Can you work these out from the model? Positions are in its coordinate system, mm. A direction names the side the tool comes from. Coordinates: 2 decimals unless noted, no trailing zeros. Order: outer loops, then holes, each group sorted by start corner. A loop starts at its lowest first (then second) coordinate and runs counter-clockwise, first axis right, second up. Notation, with made-up numbers: (-29, 33) -> (-7, 33) arc R16 ccw to (-7, 39) -> close; hole circle Ø8 at (-35, 42). An arc over 180 degrees is marked (long way). Answer as CSV lines item,"result".
from build123d import *

# Parameters (mm, degrees)
ESQUISSE1_R                                 = 30
BOSS_EXTRU_1_DEPTH                          = 10
CHANFREIN1_SIZE                             = 10
CHANFREIN1_SIZE_2                           = 7.002075382
COQUE2_T                                    = -1.5
ESQUISSE2_R                                 = 4.000000000000001
BOSS_EXTRU_2_DEPTH                          = 8.5
CHANFREIN2_SIZE                             = 8.5
CHANFREIN2_SIZE_2                           = 0.445466124
ESQUISSE5_R                                 = 2.5545338760941463
ENL_V_MAT_EXTRU_1_DEPTH                     = 10
R_P_TITION_CIRCULAIRE1_COUNT                = 3
CHANFREIN2_OF_R_P_TITION_CIRCULAIRE1_SIZE   = 0.445466124
CHANFREIN2_OF_R_P_TITION_CIRCULAIRE1_SIZE_2 = 8.5
ESQUISSE6_R                                 = 8.5
ENL_V_MAT_EXTRU_2_DEPTH                     = 8.5


with BuildPart() as part:
    # Esquisse1 → Boss.-Extru.1 (new body)
    with BuildSketch(Plane(origin=(0, 0, 0), x_dir=(1, 0, 0), z_dir=(0, 1, 0))):
        with Locations(Location((0, 0, 0), (0, 0, 270))):
            Circle(ESQUISSE1_R)
    extrude(amount=BOSS_EXTRU_1_DEPTH)

    # Chanfrein1
    # the kernel refuses this chamfer: 10, 7.002075382 mm, written as the material it takes off along each edge
    with BuildSketch(Plane(origin=(0, 10, 0), x_dir=(-1.8e-16, 0, 1), z_dir=(-1, 0, -1.8e-16))) as chanfrein1_piece_1:
        Polygon((30, -CHANFREIN1_SIZE), (30 - CHANFREIN1_SIZE_2, 0), (30, 0), align=None)
    revolve(axis=Axis((0, 10, 0), (0, 1, 0)), mode=Mode.SUBTRACT)

    # Coque2
    coque2_openings = [part.faces().sort_by_distance(p)[0] for p in [
        (0, 0, 0),
    ]]
    offset(amount=COQUE2_T, openings=coque2_openings, kind=Kind.INTERSECTION)

    # Esquisse2 → Boss.-Extru.2 (add)
    with BuildSketch(Plane.XZ.offset(-8.5)):
        with Locations(Location((-16, 0, 0), (0, 0, 90))):
            Circle(ESQUISSE2_R)
    boss_extru_2 = extrude(amount=BOSS_EXTRU_2_DEPTH)

    # Chanfrein2
    # the kernel refuses this chamfer: 8.5, 0.445466124 mm, written as the material it takes off along each edge
    with BuildSketch(Plane(origin=(-16, 0, 0), x_dir=(0, 0, 1), z_dir=(1, 0, 0))) as chanfrein2_piece_1_section:
        Polygon((4.000000000000001, -CHANFREIN2_SIZE), (4.000000000000001 - CHANFREIN2_SIZE_2, 0), (4.000000000000001, 0), align=None)
    chanfrein2_piece_1 = revolve(axis=Axis((-16, 0, 0), (0, -1, 0)), mode=Mode.PRIVATE)
    chanfrein2_piece_1 = split(chanfrein2_piece_1, bisect_by=Plane(origin=(-16, 8.5, -3.8124488578332274), z_dir=(0, -1, 0)), keep=Keep.TOP, mode=Mode.PRIVATE)
    add(chanfrein2_piece_1, mode=Mode.SUBTRACT)

    # Esquisse5 → Enlèv. mat.-Extru.1 (cut)
    with BuildSketch(Plane.XZ):
        with Locations(Location((-16, 0, 0), (0, 0, 270))):
            Circle(ESQUISSE5_R)
    enl_v_mat_extru_1 = extrude(amount=-ENL_V_MAT_EXTRU_1_DEPTH, mode=Mode.SUBTRACT)

    # Répétition circulaire1: Boss.-Extru.2, Enlèv. mat.-Extru.1 ×3 about axis
    r_p_tition_circulaire1_axis = Axis((9.3e-16, 0, 6.2e-16), (0, 1, 0))
    add([boss_extru_2.rotate(r_p_tition_circulaire1_axis, i * 360 / R_P_TITION_CIRCULAIRE1_COUNT) for i in range(1, R_P_TITION_CIRCULAIRE1_COUNT)])
    add([enl_v_mat_extru_1.rotate(r_p_tition_circulaire1_axis, i * 360 / R_P_TITION_CIRCULAIRE1_COUNT) for i in range(1, R_P_TITION_CIRCULAIRE1_COUNT)], mode=Mode.SUBTRACT)

    # Chanfrein2 of Répétition circulaire1
    # the kernel refuses this chamfer: 8.5, 0.445466124 mm, written as the material it takes off along each edge
    with BuildSketch(Plane(origin=(7.999999999999997, 0, 13.856406460551021), x_dir=(0.8660254037844387, 0, -0.5000000000000001), z_dir=(-0.5000000000000001, 0, -0.8660254037844387))) as chanfrein2_of_r_p_tition_circulaire1_piece_1_section:
        Polygon((4 - CHANFREIN2_OF_R_P_TITION_CIRCULAIRE1_SIZE, 0), (4.000000000000002, -CHANFREIN2_OF_R_P_TITION_CIRCULAIRE1_SIZE_2), (4, 0), align=None)
    chanfrein2_of_r_p_tition_circulaire1_piece_1 = revolve(axis=Axis((7.999999999999997, 0, 13.856406460551021), (0, -1, 0)), mode=Mode.PRIVATE)
    chanfrein2_of_r_p_tition_circulaire1_piece_1 = split(chanfrein2_of_r_p_tition_circulaire1_piece_1, bisect_by=Plane(origin=(4.6983224384874545, 8.5, 15.762630889467637), z_dir=(0, -1, 0)), keep=Keep.TOP, mode=Mode.PRIVATE)
    add(chanfrein2_of_r_p_tition_circulaire1_piece_1, mode=Mode.SUBTRACT)
    with BuildSketch(Plane(origin=(8.000000000000009, 0, -13.856406460551014), x_dir=(-0.8660254037844384, 0, -0.5000000000000003), z_dir=(-0.5000000000000003, 0, 0.8660254037844384))) as chanfrein2_of_r_p_tition_circulaire1_piece_2_section:
        Polygon((4 - CHANFREIN2_OF_R_P_TITION_CIRCULAIRE1_SIZE, 0), (4, -CHANFREIN2_OF_R_P_TITION_CIRCULAIRE1_SIZE_2), (4, 0), align=None)
    chanfrein2_of_r_p_tition_circulaire1_piece_2 = revolve(axis=Axis((8.000000000000009, 0, -13.856406460551014), (0, -1, 0)), mode=Mode.PRIVATE)
    chanfrein2_of_r_p_tition_circulaire1_piece_2 = split(chanfrein2_of_r_p_tition_circulaire1_piece_2, bisect_by=Plane(origin=(11.301677561512552, 8.5, -11.950182031634398), z_dir=(0, -1, 0)), keep=Keep.TOP, mode=Mode.PRIVATE)
    add(chanfrein2_of_r_p_tition_circulaire1_piece_2, mode=Mode.SUBTRACT)

    # Esquisse6 → Enlèv. mat.-Extru.2 (cut)
    with BuildSketch(Plane.XZ.offset(-8.5)):
        with Locations(Location((0, 0, 0), (0, 0, 270))):
            Circle(ESQUISSE6_R)
    extrude(amount=-ENL_V_MAT_EXTRU_2_DEPTH, mode=Mode.SUBTRACT)


solid = part.part
Q1. We'd pull the mould along Z, two halves only. Please class faces 1 (the conical face through (-12.65, 4.19, 1.74)), 2 (the flat face through (0, 10, 10)), 3 (the conical face through (7.01, 9.514, 22.26)): pulls with the +Z half, pulls with the -Z half, needs draft (parallel to the pull), parting line crosses it, or undercut.
Solution:
face 1,"undercut"
face 2,"needs draft"
face 3,"parting line crosses it"
Q2. Imagine slicing it at A-A (x = 0). List the corners of the cut face in (y, z) for me, and give its area (3 significant figures).
Solution:
outline,"(0, -30) -> (10, -23) -> (10, -8.5) -> (8.5, -8.5) -> (8.5, -22.22) -> (0, -28.17) -> close; (0, 28.17) -> (8.5, 22.22) -> (8.5, 8.5) -> (10, 8.5) -> (10, 23) -> (0, 30) -> close"
area,"76.2 mm2"
Q3. Imagine slicing it at C-C (y = 4.25). List the corners of the cut face in (x, z) for me, and give its area (3 significant figures).
Solution:
outline,"circle Ø54.05 at (0, 0); circle Ø7.55 at (-16, 0); circle Ø7.55 at (8, -13.86); circle Ø7.55 at (8, 13.86); hole circle Ø50.39 at (0, 0); hole circle Ø5.11 at (-16, 0); hole circle Ø5.11 at (8, -13.86); hole circle Ø5.11 at (8, 13.86)"
area,"373 mm2"
Q4. Imagine slicing it at D-D (y = 0.75). List the corners of the cut face in (x, z) for me, and give its area (3 significant figures).
Solution:
outline,"circle Ø58.95 at (0, 0); circle Ø7.19 at (-16, 0); circle Ø7.19 at (8, -13.86); circle Ø7.19 at (8, 13.86); hole circle Ø55.29 at (0, 0); hole circle Ø5.11 at (-16, 0); hole circle Ø5.11 at (8, -13.86); hole circle Ø5.11 at (8, 13.86)"
area,"389 mm2"
Q5. Imagine slicing it at B-B (z = 0). List the corners of the cut face in (x, y) for me, and give its area (3 significant figures).
Solution:
outline,"(-30, 0) -> (-28.17, 0) -> (-22.22, 8.5) -> (-20, 8.5) -> (-19.55, 0) -> (-18.55, 0) -> (-18.55, 10) -> (-23, 10) -> close; (-13.45, 0) -> (-12.45, 0) -> (-12, 8.5) -> (-8.5, 8.5) -> (-8.5, 10) -> (-13.45, 10) -> close; (8.5, 8.5) -> (22.22, 8.5) -> (28.17, 0) -> (30, 0) -> (23, 10) -> (8.5, 10) -> close"
area,"89.3 mm2"
Q6. Which directions (+Z, -Z, +X, -X, +Y, -Y) give clear straight access to the entire face, cutting with the end or side of a thin tool? Please do faces 4 (the flat face through (0, 8.5, 10)), 5 (the flat face through (6, 0, 16)).
Solution:
face 4,"-Y"
face 5,"+Z, -Z, +X, -X, -Y"
Q7. If I drill on line 1 (X direction, y = 0.5, z = 14.5); line 2 (Z direction, x = 4.5, y = 8); line 3 (X direction, y = 4, z = -11), over which ranges is the centre line in solid material (lowest first)?
Solution:
line 1,"-25.86 to -23.74, 4.48 to 5.53, 10.47 to 11.52, 23.74 to 25.86"
line 2,"-23.98 to -22.11, -15.74 to -11.97, 11.97 to 15.74, 22.11 to 23.98"
line 3,"-24.88 to -22.86, 5.55 to 10.45, 22.86 to 24.88"
Q8. For P1, Ø3, axis at x = -16, z = 0, coming from the -Y side; P2, Ø4, axis at x = 8.5, z = 0, coming from the -Y side; P3, Ø4, axis at x = 11.5, y = 8, coming from the +Z side; P4, Ø8, axis at x = -2.5, z = 21, coming from the -Y side, each with a flat end and sliding along its axis, tell me the tip position at first contact or that it passes through.
Solution:
P1,"through"
P2,"y = 8.5"
P3,"z = 23.36"
P4,"y = 4.31"
